from build123d import *

# Parameters (mm, degrees)
BOSS_EXTRUDE1_DEPTH = 5
CUT_EXTRUDE1_DEPTH  = 43.720018727
FILLET1_R           = 2.54
SKETCH9_W           = 20
SKETCH9_H           = 5.200996356
BOSS_EXTRUDE5_DEPTH = 33.75
SKETCH11_W          = 3.25
SKETCH11_H          = 1.5
BOSS_EXTRUDE6_DEPTH = 15
SKETCH12_R          = 5.5
CUT_EXTRUDE3_DEPTH  = 70.655258104
FILLET3_R           = 2.54


with BuildPart() as part:
    # Sketch1 → Boss-Extrude1 (new body)
    with BuildSketch(Plane(origin=(0, 0, 0), x_dir=(1, 0, 0), z_dir=(0, 1, 0))):
        Polygon((-30, -10), (-30, -30), (30, -30), (30, -10), (10, -10), (10, 10), (30, 10), (30, 30), (-30, 30), (-30, 10), (-10, 10), (-10, -10), align=None)
    extrude(amount=BOSS_EXTRUDE1_DEPTH)

    # Sketch2 → Cut-Extrude1 (cut, through all)
    with BuildSketch(Plane(origin=(0, 5, 0), x_dir=(1, 0, 0), z_dir=(0, 1, 0))):
        with BuildLine():
            Line((-18.55, 18.5), (18.55, 18.5))
            ThreePointArc((18.55, 18.5), (19.575304833, 18.924695167), (20, 19.95))
            Line((20, 19.95), (20, 20.05))
            ThreePointArc((20, 20.05), (19.575304833, 21.075304833), (18.55, 21.5))
            Line((18.55, 21.5), (-18.55, 21.5))
            ThreePointArc((-18.55, 21.5), (-19.575304833, 21.075304833), (-20, 20.05))
            Line((-20, 20.05), (-20, 19.95))
            ThreePointArc((-20, 19.95), (-19.575304833, 18.924695167), (-18.55, 18.5))
        make_face()
        with BuildLine():
            Line((-18.55, -21.5), (18.55, -21.5))
            ThreePointArc((18.55, -21.5), (19.575304833, -21.075304833), (20, -20.05))
            Line((20, -20.05), (20, -19.95))
            ThreePointArc((20, -19.95), (19.575304833, -18.924695167), (18.55, -18.5))
            Line((18.55, -18.5), (-18.55, -18.5))
            ThreePointArc((-18.55, -18.5), (-19.575304833, -18.924695167), (-20, -19.95))
            Line((-20, -19.95), (-20, -20.05))
            ThreePointArc((-20, -20.05), (-19.575304833, -21.075304833), (-18.55, -21.5))
        make_face()
    extrude(amount=-CUT_EXTRUDE1_DEPTH, mode=Mode.SUBTRACT)

    # Fillet1
    fillet1_edges = [part.edges().sort_by_distance(p)[0] for p in [
        (-10, 2.5, -10),
        (-30, 2.5, -10),
        (-30, 2.5, -30),
        (30, 2.5, -30),
        (30, 2.5, -10),
        (10, 2.5, -10),
        (10, 2.5, 10),
        (30, 2.5, 10),
        (30, 2.5, 30),
        (-30, 2.5, 30),
        (-30, 2.5, 10),
        (-10, 2.5, 10),
    ]]
    fillet(fillet1_edges, radius=FILLET1_R)

    # Sketch9 → Boss-Extrude5 (add)
    with BuildSketch(Plane(origin=(0, 5, 0), x_dir=(1, 0, 0), z_dir=(0, 1, 0))):
        Rectangle(SKETCH9_W, SKETCH9_H)
    extrude(amount=BOSS_EXTRUDE5_DEPTH)

    # Sketch11 → Boss-Extrude6 (add)
    with BuildSketch(Plane(origin=(0, 38.75, 0), x_dir=(1, 0, 0), z_dir=(0, 1, 0))):
        Polygon((-10, 2.600498178), (-10, 0.75), (-6.75, 0.75), (6.75, 0.75), (10, 0.75), (10, 2.600498178), align=None)
        with Locations((-8.375, 0)):
            Rectangle(SKETCH11_W, SKETCH11_H)
        Polygon((-6.75, -0.75), (-10, -0.75), (-10, -2.600498178), (10, -2.600498178), (10, -0.75), (6.75, -0.75), align=None)
        with Locations((8.375, 0)):
            Rectangle(SKETCH11_W, SKETCH11_H)
    extrude(amount=BOSS_EXTRUDE6_DEPTH)

    # Sketch12 → Cut-Extrude3 (cut, through all)
    with BuildSketch(Plane.XY.offset(2.600498178)):
        with Locations((0, 45)):
            Circle(SKETCH12_R)
    extrude(amount=-CUT_EXTRUDE3_DEPTH, mode=Mode.SUBTRACT)

    # Fillet3
    fillet3_edges = [part.edges().sort_by_distance(p)[0] for p in [
        (0, 5, -2.600498178),
        (0, 5, 2.600498178),
        (10, 53.75, 0),
        (-10, 53.75, 0),
    ]]
    fillet(fillet3_edges, radius=FILLET3_R)


solid = part.part
Geometry: final body of the model. Coordinates: model frame, mm. A direction names the side the tool comes from. Round coordinates to 2 decimals unless told otherwise and drop trailing zeros. Loops run counter-clockwise (first coordinate to the right, second up) from the corner with the lowest first, then second, coordinate; pieces in that order, holes last.
Q1. Pin query (flat end, axial travel): P1, Ø16, axis at x = -3.5, y = 32.5, coming from the -Z side; P2, Ø0.8, axis at y = 45, z = 0, coming from the -X side; P3, Ø3, axis at y = 6, z = 1.5, coming from the +X side; P4, Ø9, axis at x = 0, y = 45, coming from the -Z side. Return the tip coordinate at first contact, or that it passes through.
Q2. Section A-A on x = -21. Return loops of the section in (y, z), plus the area to 3 significant figures.
Q3. Access query for faces 4 (the flat face through (0, 51, -0.75)), 5 (the flat face through (-20, 2, -10)), 6 (the flat face through (0, 5, -18)), 7 (the flat face through (0, 3, -18.5)), 8 (the flat face through (20, 2, -10)). Directions: +Z, -Z, +X, -X, +Y, -Y. A direction counts if a zero-diameter tool reaches every point of the face in a straight line with its end or side. Return the directions, or none.
Q4. Material intervals for L1, parallel to Y at x = 0, z = 1.25; L2, parallel to X at y = 41.5, z = 0.5; L3, parallel to Y at x = -2, z = 17, sorted ascending.
Q5. Section B-B on x = 0. State how many separate pieces and enclosed holes the cut face has, plus the area to 3 significant figures.
Q6. Section C-C on y = 45. Return loops of the section in (x, z), plus the area to 3 significant figures.
Q7. Section D-D on z = 25. Return loops of the section in (x, y), plus the area to 3 significant figures.
Q8. Pull-direction query (Y, two-part tool) for faces 1 (the cylindrical face through (-10.724, 2.535, -9.236)), 2 (the cylindrical face through (-0.716, 50.453, -1.662)), 3 (the cylindrical face through (0.14, 5.764, 3.325)); classes: released by +Y, released by -Y, zero draft, split by the parting line, or undercut.
Evaluation:
1. P1: stops at z = -2.6
1. P2: stops at x = -10
1. P3: stops at x = 10
1. P4: passes through
2. outline: (0, -30) - (5, -30) - (5, -10) - (0, -10) - close; (0, 10) - (5, 10) - (5, 30) - (0, 30) - close
2. area: 200 mm2
3. face 4: +Y
3. face 5: -X, +Y, -Y
3. face 6: -Z, +X, -X, +Y
3. face 7: +Y, -Y
3. face 8: +X, +Y, -Y
4. L1: y = 0 to 39.5, 50.5 to 53.75
4. L2: x = -10 to -6.75, 6.75 to 10
4. L3: y = 0 to 5
5. separate pieces: 5
5. enclosed holes: 0
5. area: 463 mm2
6. outline: (-10, -2.6) - (-5.5, -2.6) - (-5.5, -0.75) - (-6.75, -0.75) - (-6.75, 0.75) - (-5.5, 0.75) - (-5.5, 2.6) - (-10, 2.6) - close; (5.5, -2.6) - (10, -2.6) - (10, 2.6) - (5.5, 2.6) - (5.5, 0.75) - (6.75, 0.75) - (6.75, -0.75) - (5.5, -0.75) - close
6. area: 43.1 mm2
7. outline: (-30, 0) - (30, 0) - (30, 5) - (-30, 5) - close
7. area: 300 mm2
8. face 1: zero draft
8. face 2: undercut
8. face 3: released by +Y
